from build123d import *

# Parameters (mm, degrees)
SKETCH1_W           = 100
SKETCH1_H           = 49.852187789
BOSS_EXTRUDE3_DEPTH = 150
SKETCH2_R           = 47.5
CUT_EXTRUDE1_DEPTH  = 140
CUT_EXTRUDE1_DRAFT  = -2


with BuildPart() as part:
    # Sketch1 → Boss-Extrude3 (new body)
    with BuildSketch(Plane(origin=(0, 0, 0), x_dir=(1, 0, 0), z_dir=(0, 1, 0))):
        with Locations((0, 25.073906106)):
            Rectangle(SKETCH1_W, SKETCH1_H)
    extrude(amount=BOSS_EXTRUDE3_DEPTH)


with BuildPart() as cut_extrude1_tool:
    # Sketch2 → Cut-Extrude1 (with draft: the straight prism first)
    with BuildSketch(Plane.XZ):
        Circle(SKETCH2_R)
    extrude(amount=-CUT_EXTRUDE1_DEPTH)
    # Cut-Extrude1: the draft: its side faces are tilted about the plane it starts from
    cut_extrude1_sides = [cut_extrude1_tool.faces().sort_by_distance(p)[0] for p in [
        (-47.5, 70, 0),
    ]]
    draft(cut_extrude1_sides, Plane.XZ, CUT_EXTRUDE1_DRAFT)


with BuildPart() as part_1:
    add(part.part)

    # Cut-Extrude1: cut by cut_extrude1_tool
    add(cut_extrude1_tool.part, mode=Mode.SUBTRACT)


solid = part_1.part
Verification items for the finished model (mm, model axes). Round coordinates to 2 decimals unless told otherwise and drop trailing zeros. Write each loop counter-clockwise with the first axis right and the second up, starting at its lowest first coordinate (ties: lowest second). Pieces come first, ordered by that corner, then holes.
(1) Material ranges on line 1 (Y direction, x = -15.5, z = -36.5); line 2 (X direction, y = 42, z = -38); line 3 (X direction, y = 20, z = -16.5), recorded low to high.
Returned:
line 1: y = 140 to 150
line 2: x = -50 to -25.98, 25.98 to 50
line 3: x = -50 to -43.8, 43.8 to 50
(2) Mould release check, pull along X, two halves, no side actions. Record for faces 1 (the flat face through (-50, 74, -25)), 2 (the flat face through (-1, 140, -16)), 3 (the conical face through (-0.99, 69.02, -45.08)), 4 (the flat face through (50, 74, -25)): pulls with the +X half, pulls with the -X half, needs draft (parallel to the pull), parting line crosses it, or undercut.
Returned:
face 1: pulls with the -X half
face 2: undercut
face 3: undercut
face 4: pulls with the +X half
(3) Depth check by flat-ended pin: pin 1 Ø8 at (x, z) = (14.5, -27.5) entering from -Y; pin 2 Ø3 at (x, y) = (-21.5, 82.5) entering from +Z. Enter the tip coordinate at first touch or a pass-through.
Returned:
pin 1: stops at y = 140
pin 2: stops at z = -38.23
(4) Section check A-A (x = 0). Enter the section's corners in (y, z), plus the area to 3 significant figures.
Returned:
outline: (0, -50) - (150, -50) - (150, -0.15) - (140, -0.15) - (140, -42.61) - (0, -47.5) - close
area: 1,190 mm2
